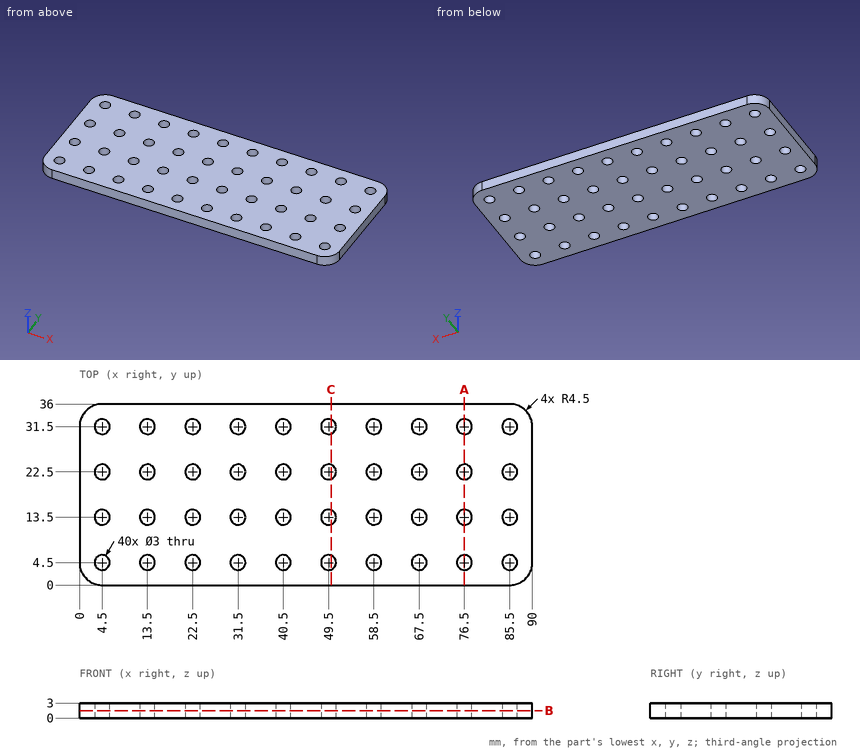
For this review, use the dimensioned drawing (mm, ordinates from the lowest corner) and the shaded views. Round coordinates to 2 decimals unless told otherwise and drop trailing zeros. Loops run counter-clockwise (first coordinate to the right, second up) from the corner with the lowest first, then second, coordinate; pieces in that order, holes last. Notation, with made-up numbers: (-18, 81) -> (-10, 81) arc R14 cw to (-10, 99) -> close; hole circle Ø5 at (71.5, -32.5). An arc over 180 degrees is marked (long way). Write item = value, one per line. Start each with the question number.
Item 1: To check wall thickness, follow L1, parallel to Y at x = 13.5, z = 1.1; L2, parallel to Y at x = 86, z = 0.55. State the ranges of each line that lie inside material, in increasing order.
Item 2: Take a section at C-C on x = 50. Give the boundary of the cut face in (y, z), plus the area to 3 significant figures.
Item 3: Take a section at A-A on x = 76.5. Give the boundary of the cut face in (y, z).
Item 4: Insertion check: pin 1 (4 mm diameter, centred on x = 22.5, y = 22.5, fed in from -Z). The pin has a flat end and moves straight along its axis. Give the tip position at first contact, or say it passes through.
Item 5: Take a section at B-B on z = 1.5. Count the separate pieces of the cut face and the enclosed holes in it, plus the area to 3 significant figures.
Result:
q1.L1 = 0 to 3, 6 to 12, 15 to 21, 24 to 30, 33 to 36
q1.L2 = 0.03 to 3.09, 5.91 to 12.09, 14.91 to 21.09, 23.91 to 30.09, 32.91 to 35.97
q2.outline = (0, 0) -> (3.09, 0) -> (3.09, 3) -> (0, 3) -> close; (5.91, 0) -> (12.09, 0) -> (12.09, 3) -> (5.91, 3) -> close; (14.91, 0) -> (21.09, 0) -> (21.09, 3) -> (14.91, 3) -> close; (23.91, 0) -> (30.09, 0) -> (30.09, 3) -> (23.91, 3) -> close; (32.91, 0) -> (36, 0) -> (36, 3) -> (32.91, 3) -> close
q2.area = 74.1 mm²
q3.outline = (0, 0) -> (3, 0) -> (3, 3) -> (0, 3) -> close; (6, 0) -> (12, 0) -> (12, 3) -> (6, 3) -> close; (15, 0) -> (21, 0) -> (21, 3) -> (15, 3) -> close; (24, 0) -> (30, 0) -> (30, 3) -> (24, 3) -> close; (33, 0) -> (36, 0) -> (36, 3) -> (33, 3) -> close
q4.pin_1 = 0
q5.separate_pieces = 1
q5.enclosed_holes = 40
q5.area = 2,940 mm²
